```python
from build123d import *

# Parameters (mm, degrees)
F0_R     = 6.0638349588
F0_R_2   = 5.3684107219
F0_R_3   = 5.8892395432
F1_DEPTH = 38.1
F2_W     = 23.8111317158
F2_H     = 9.7214011475
F3_DEPTH = 55.1676675677
F4_W     = 9.6149358433
F4_H     = 3.907698667
F5_DEPTH = 82.5948805938


with BuildPart() as f1:
    # F0 (on Top) → F1 (new body)
    with BuildSketch(Plane.XY):
        Polygon((33.8834859431, 24.6326997876), (-48.7103946507, 24.6326997876), (-48.7103946507, -30.5349677801), (-5.2067479119, -30.5349677801), (-5.2067479119, -21.3928986341), (33.8834859431, -21.3928986341), align=None)
        with Locations((4.881054163, -8.1526581198)):
            Circle(F0_R, mode=Mode.SUBTRACT)
        with Locations((22.8499509394, -7.206926588)):
            Circle(F0_R_2, mode=Mode.SUBTRACT)
        with Locations((5.5115413852, 15.1753844693)):
            Circle(F0_R_3, mode=Mode.SUBTRACT)
        with Locations((21.5889755636, 14.860141091)):
            Circle(F0_R_3, mode=Mode.SUBTRACT)
    extrude(amount=F1_DEPTH)

    # F2 (on face) → F3 (cut, through all)
    with BuildSketch(Plane(origin=(0, 24.6326997876, 0), x_dir=(-1, 0, 0), z_dir=(0, 1, 0))):
        Polygon((-33.8834859431, 0), (16.8716572225, 38.1), (-33.8834859431, 38.1), align=None)
        with Locations((36.8048287928, 4.8607005738)):
            Rectangle(F2_W, F2_H)
    extrude(amount=-F3_DEPTH, mode=Mode.SUBTRACT)

    # F4 (on face) → F5 (cut, through all)
    with BuildSketch(Plane(origin=(-48.7103946507, 0, 0), x_dir=(0, -1, 0), z_dir=(-1, 0, 0))):
        with Locations((2.5730371708, 36.1461506665)):
            Rectangle(F4_W, F4_H)
    extrude(amount=-F5_DEPTH, mode=Mode.SUBTRACT)


solid = f1.part
```
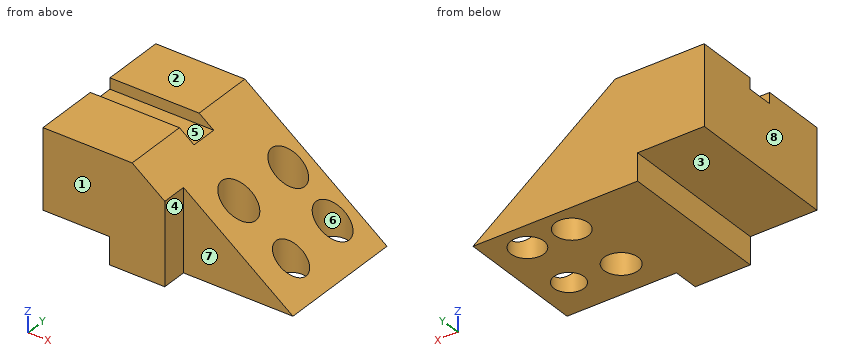
The model under review builds one solid part; all positions refer to its coordinate system, in mm. Face numbers are marked on the shaded views. A direction names the side the tool comes from. Give positions to 0.01 mm unless a question says otherwise; leave off trailing zeros. Write each loop counter-clockwise with the first axis right and the second up, starting at its lowest first coordinate (ties: lowest second). Pieces come first, ordered by that corner, then holes. Notation, with made-up numbers: M 44.25,51.25 L 79.25,51.25 A13 ccw 79.25,70.25 Z; hole C 30.25,-14.75 d6. An arc over 180 degrees is marked long. Answer in a Markdown table with one row per item.
Item 1: For line 1 along X through (y, z) = (13, 2.5); line 2 along Y through (x, z) = (-33, 35.5); line 3 along Y through (x, z) = (-3.5, 23.5), list the stretches that pass through material, from the lowest coordinate up.
Check sheet entries:
| item | result |
|---|---|
| line 1 | -24.9 to 0.04, 10.98 to 16, 27.18 to 30.55 |
| line 2 | -30.53 to -7.38, 2.23 to 24.63 |
| line 3 | -21.39 to 24.63 |
Item 2: Draft analysis for pull direction X (two halves, no side actions). For the marked faces 6, 7 and 8, state which applies: +X half, -X half, draft (parallel to the pull), parting line (faces both ways), or undercut.
Check sheet entries:
| item | result |
|---|---|
| face 6 | undercut |
| face 7 | draft |
| face 8 | -X half |
Item 3: Add section B-B on y = -11.5. Give the boundary of the cut face in (x, z).
Check sheet entries:
| item | result |
|---|---|
| outline | M -48.71,9.72 L -24.9,9.72 L -24.9,0 L -0.18,0 L -0.18,25.57 L -16.87,38.1 L -48.71,38.1 Z; M 9.94,0 L 19.63,0 L 19.63,10.7 L 9.94,17.98 Z; M 26.07,0 L 33.88,0 L 26.07,5.86 Z |
Item 4: Add section A-A on x = -21.5. Give the boundary of the cut face in (y, z).
Check sheet entries:
| item | result |
|---|---|
| outline | M -30.53,0 L 24.63,0 L 24.63,38.1 L 2.23,38.1 L 2.23,34.19 L -7.38,34.19 L -7.38,38.1 L -30.53,38.1 Z |
Item 5: For P1, Ø8, axis at y = -6, z = 3, coming from the -X side; P2, Ø1.5, axis at x = -9, y = -23.5, coming from the +Z side; P3, Ø4.5, axis at y = -28, z = 17.5, coming from the +X side, all flat-tipped, find the tip position at first contact; note any pin that passes through.
Check sheet entries:
| item | result |
|---|---|
| P1 | x = -24.9 |
| P2 | z = 32.75 |
| P3 | x = -5.21 |
Item 6: Add section C-C on x = 20. Give the boundary of the cut face in (y, z).
Check sheet entries:
| item | result |
|---|---|
| outline | M -21.39,0 L -11.76,0 L -11.76,10.42 L -21.39,10.42 Z; M -2.66,0 L 9.19,0 L 9.19,10.42 L -2.66,10.42 Z; M 20.53,0 L 24.63,0 L 24.63,10.42 L 20.53,10.42 Z |
Item 7: Add section D-D on z = 24. Give the boundary of the cut face in (x, y), plus the area to 3 significant figures.
Check sheet entries:
| item | result |
|---|---|
| outline | M -48.71,-30.53 L -5.21,-30.53 L -5.21,-21.39 L 1.91,-21.39 L 1.91,-13.44 A6.06 cw 1.91,-2.87 L 1.91,10.51 A5.89 cw 1.91,19.84 L 1.91,24.63 L -48.71,24.63 Z |
| area | 2,690 mm2 |
Item 8: Tool access review of the marked faces 1, 2, 3, 4 and 5: name each direction out of +Z, -Z, +X, -X, +Y, -Y from which nothing blocks a thin tool from reaching the whole face with its end or side.
Check sheet entries:
| item | result |
|---|---|
| face 1 | +Z, -Z, +X, -X, -Y |
| face 2 | +Z, +X, -X, +Y, -Y |
| face 3 | -Z, -X, +Y, -Y |
| face 4 | +Z, -Z, +X, -Y |
| face 5 | +Z, +X, -X |
